```python
from build123d import *

# Parameters (mm, degrees)
SKETCH_1_W      = 20.32
SKETCH_1_H      = 8.5
EXTRUDE_1_DEPTH = 2.5
SKETCH_2_W      = 0.6
SKETCH_2_H      = 0.4
EXTRUDE_2_DEPTH = 3


with BuildPart() as part:
    # Эскиз1 → Бобышка-Вытянуть1 (new body)
    with BuildSketch(Plane(origin=(0, 0, 0), x_dir=(1, 0, 0), z_dir=(0, 1, 0))):
        Rectangle(SKETCH_1_W, SKETCH_1_H)
    extrude(amount=EXTRUDE_1_DEPTH)

    # Эскиз2 → Бобышка-Вытянуть2 (add)
    with BuildSketch(Plane.XY.offset(4.25)):
        with Locations((-6.35, 1.25)):
            Rectangle(SKETCH_2_W, SKETCH_2_H)
        with Locations((-8.89, 1.25)):
            Rectangle(SKETCH_2_W, SKETCH_2_H)
        with Locations((-3.81, 1.25)):
            Rectangle(SKETCH_2_W, SKETCH_2_H)
        with Locations((-1.27, 1.25)):
            Rectangle(SKETCH_2_W, SKETCH_2_H)
        with Locations((1.27, 1.25)):
            Rectangle(SKETCH_2_W, SKETCH_2_H)
        with Locations((3.81, 1.25)):
            Rectangle(SKETCH_2_W, SKETCH_2_H)
        with Locations((6.35, 1.25)):
            Rectangle(SKETCH_2_W, SKETCH_2_H)
        with Locations((8.89, 1.25)):
            Rectangle(SKETCH_2_W, SKETCH_2_H)
    extrude(amount=EXTRUDE_2_DEPTH)


solid = part.part
```
Geometry: final body of the model. Coordinates: model frame, mm. Coordinates: 2 decimals unless noted, no trailing zeros. Order: outer loops, then holes, each group sorted by start corner. A loop starts at its lowest first (then second) coordinate and runs counter-clockwise, first axis right, second up. Notation, with made-up numbers: M 12,66.25 L 65,66.25 A16 cw 65,91.25 Z; hole C 53.25,-22 d10. An arc over 180 degrees is marked long. Answer in a Markdown table with one row per item. Add a question column.
Q1. Section query C-C on y = 0.7. Return the cut outline in (x, z), and give its area (3 significant figures).
Q2. Contact query for flat-ended pins moving along their axis: P1, Ø0.5, axis at x = -6.5, z = 6, coming from the -Y side; P2, Ø0.5, axis at x = 6.5, z = 6.5, coming from the +Y side; P3, Ø1, axis at y = 1, z = 5.5, coming from the +X side. Output: stop coordinate, or through.
Q3. Section query A-A on z = 5. Count the separate pieces of the cut face and the enclosed holes in it, and give its area (3 significant figures).
Q4. Section query B-B on x = -0.25. Return the cut outline in (y, z), and give its area (4 significant figures).
Q5. Line query: L1, parallel to Y at x = -1.25, z = 4.75; L2, parallel to Z at x = 1.75, y = 1.1. Output: solid intervals per line, ascending.
Completed:
| question | item | result |
|---|---|---|
| 1 | outline | M -10.16,-4.25 L 10.16,-4.25 L 10.16,4.25 L -10.16,4.25 Z |
| 1 | area | 173 mm2 |
| 2 | P1 | stops at y = 1.05 |
| 2 | P2 | stops at y = 1.45 |
| 2 | P3 | stops at x = 9.19 |
| 3 | separate pieces | 8 |
| 3 | enclosed holes | 0 |
| 3 | area | 1.92 mm2 |
| 4 | outline | M 0,-4.25 L 2.5,-4.25 L 2.5,4.25 L 0,4.25 Z |
| 4 | area | 21.25 mm2 |
| 5 | L1 | y = 1.05 to 1.45 |
| 5 | L2 | z = -4.25 to 4.25 |
